Autodesk Fusion 360 part; units mm, degrees
sketch "Esquisse1" plane through (0, 0, 0) normal (0, 1, 0) x (1, 0, 0)
  line L0 (-367.4671, -125) -> (350, -125) construction
  arc A0 (209.2489, -218.6842) -> (223.8346, -225) centre (223.8346, -205) ccw
  arc A1 (-223.8346, -225) -> (-209.2489, -218.6842) centre (-223.8346, -205) ccw
  arc A2 (209.2489, -218.6842) -> (-209.2489, -218.6842) centre (0, -415) ccw
  line L1 (-305, 225) -> (305, 225)
  line L2 (325, 205) -> (325, -205)
  line L3 (305, -225) -> (223.8346, -225)
  line L4 (-325, -205) -> (-325, 205)
  arc A3 (325, 205) -> (305, 225) centre (305, 205) ccw
  line L5 (325, 225) -> (-325, -225) construction
  arc A4 (-305, 225) -> (-325, 205) centre (-305, 205) ccw
  arc A5 (-325, -205) -> (-305, -225) centre (-305, -205) ccw
  line L6 (-305, -225) -> (-223.8346, -225)
  line L7 (-325, 225) -> (325, -225) construction
  arc A6 (305, -225) -> (325, -205) centre (305, -205) ccw
  line L8 (215, -225) -> (325, -225)
  point P0 (-215, -225)
  dimension "d12" = 650
  dimension "d13" = 450
  dimension "d14" = 110
  dimension "d15" = 110
  dimension "d16" = 100
  dimension "d20" = 190
  dimension "d21" = 20
extrude "Extrusion1" add sketch "Esquisse1" along normal blind 3
sketch "Esquisse2" plane through (0, 3, 0) normal (0, 1, 0) x (-1, 0, 0)
  arc A0 (325, 205) -> (305, 225) centre (305, 205) ccw
  line L0 (305, 225) -> (223.8346, 225)
  arc A1 (223.8346, 225) -> (209.2489, 218.6842) centre (223.8346, 205) ccw
  arc A2 (-209.2489, 218.6842) -> (209.2489, 218.6842) centre (0, 415) ccw
  arc A3 (-209.2489, 218.6842) -> (-223.8346, 225) centre (-223.8346, 205) ccw
  line L1 (-223.8346, 225) -> (-305, 225)
  arc A4 (-305, 225) -> (-325, 205) centre (-305, 205) ccw
  line L2 (-325, 205) -> (-325, -205)
  arc A5 (-325, -205) -> (-305, -225) centre (-305, -205) ccw
  line L3 (-305, -225) -> (305, -225)
  arc A6 (305, -225) -> (325, -205) centre (305, -205) ccw
  line L4 (325, -205) -> (325, 205)
  line L5 (14.7224, 11.5) -> (0, 37)
  line L6 (-14.7224, 11.5) -> (14.7224, 11.5)
  line L7 (0, 37) -> (-14.7224, 11.5)
  line L8 (-61.5, -59.7224) -> (-61.5, -30.2776)
  line L9 (-87, -45) -> (-61.5, -59.7224)
  line L10 (-61.5, -30.2776) -> (-87, -45)
  line L11 (-14.7224, -101.5) -> (0, -127)
  line L12 (0, -127) -> (14.7224, -101.5)
  line L13 (14.7224, -101.5) -> (-14.7224, -101.5)
  line L14 (61.5, -30.2776) -> (61.5, -59.7224)
  line L15 (388.9907, -50) -> (-400, -50) construction
  line L16 (87, -45) -> (61.5, -30.2776)
  line L17 (61.5, -59.7224) -> (87, -45)
  point P0 (70, -45)
  point P1 (0, -110)
  point P2 (0, 20)
  dimension "d46" = 5
  dimension "d48" = 70
  dimension "d52" = 17
extrude "Extrusion2" cut sketch "Esquisse2" against normal blind 1 contours L5 L6 L7 | L8 L9 L10 | L11 L12 L13 | L14 L16 L17
sketch "Esquisse3" plane through (0, 3, 0) normal (0, 1, 0) x (-1, 0, 0)
  line L0 (0, -127) -> (-14.7224, -101.5)
  line L1 (-14.7224, -101.5) -> (14.7224, -101.5)
  line L2 (14.7224, -101.5) -> (0, -127)
  line L3 (-61.5, -59.7224) -> (-87, -45)
  line L4 (-87, -45) -> (-61.5, -30.2776)
  line L5 (-61.5, -30.2776) -> (-61.5, -59.7224)
  line L6 (61.5, -30.2776) -> (87, -45)
  line L7 (87, -45) -> (61.5, -59.7224)
  line L8 (61.5, -59.7224) -> (61.5, -30.2776)
  line L9 (14.7224, 11.5) -> (-14.7224, 11.5)
  line L10 (-14.7224, 11.5) -> (0, 37)
  line L11 (0, 37) -> (14.7224, 11.5)
  arc A0 (325, 205) -> (305, 225) centre (305, 205) ccw
  line L12 (305, 225) -> (223.8346, 225)
  arc A1 (223.8346, 225) -> (209.2489, 218.6842) centre (223.8346, 205) ccw
  arc A2 (-209.2489, 218.6842) -> (209.2489, 218.6842) centre (0, 415) ccw
  arc A3 (-209.2489, 218.6842) -> (-223.8346, 225) centre (-223.8346, 205) ccw
  line L13 (-223.8346, 225) -> (-305, 225)
  arc A4 (-305, 225) -> (-325, 205) centre (-305, 205) ccw
  line L14 (-325, 205) -> (-325, -205)
  arc A5 (-325, -205) -> (-305, -225) centre (-305, -205) ccw
  line L15 (-305, -225) -> (305, -225)
  arc A6 (305, -225) -> (325, -205) centre (305, -205) ccw
  line L16 (325, -205) -> (325, 205)
  line L17 (0, -325) -> (0, 225)
  line L18 (290, -225) -> (255, -260)
  line L19 (255, -260) -> (0, -260)
  line L20 (325, -175) -> (360, -140)
  line L21 (360, -140) -> (360, 140)
  line L22 (360, 140) -> (325, 175)
  line L23 (-255, -260) -> (0, -260)
  line L24 (-290, -225) -> (-255, -260)
  line L25 (-325, -175) -> (-360, -140)
  line L26 (-360, -140) -> (-360, 140)
  line L27 (-360, 140) -> (-325, 175)
  dimension "d22" = 35
  dimension "d23" = 45
  dimension "d24" = 580
  dimension "d25" = 35
  dimension "d26" = 45
  dimension "d27" = 45
  dimension "d28" = 350
  dimension "d30" = 30
extrude "Extrusion3" add sketch "Esquisse3" against normal up to surface (3 mm away) contours L15 L17 L23 L24 | L15 L17 L18 L19 | L14 L25 L26 L27 | L16 L20 L21 L22
sketch "Esquisse4" plane through (0, 3, 0) normal (0, 1, 0) x (-1, 0, 0)
  line L0 (0, -127) -> (-14.7224, -101.5)
  line L1 (-14.7224, -101.5) -> (14.7224, -101.5)
  line L2 (14.7224, -101.5) -> (0, -127)
  line L3 (-61.5, -59.7224) -> (-87, -45)
  line L4 (-87, -45) -> (-61.5, -30.2776)
  line L5 (-61.5, -30.2776) -> (-61.5, -59.7224)
  line L6 (61.5, -30.2776) -> (87, -45)
  line L7 (87, -45) -> (61.5, -59.7224)
  line L8 (61.5, -59.7224) -> (61.5, -30.2776)
  line L9 (14.7224, 11.5) -> (-14.7224, 11.5)
  line L10 (-14.7224, 11.5) -> (0, 37)
  line L11 (0, 37) -> (14.7224, 11.5)
  arc A0 (325, 205) -> (305, 225) centre (305, 205) ccw
  line L12 (305, 225) -> (223.8346, 225)
  arc A1 (223.8346, 225) -> (209.2489, 218.6842) centre (223.8346, 205) ccw
  arc A2 (-209.2489, 218.6842) -> (209.2489, 218.6842) centre (0, 415) ccw
  arc A3 (-209.2489, 218.6842) -> (-223.8346, 225) centre (-223.8346, 205) ccw
  line L13 (-223.8346, 225) -> (-305, 225)
  arc A4 (-305, 225) -> (-325, 205) centre (-305, 205) ccw
  line L14 (-325, 205) -> (-325, 175)
  line L15 (-325, 175) -> (-360, 140)
  line L16 (-360, 140) -> (-360, -140)
  line L17 (-360, -140) -> (-325, -175)
  line L18 (-325, -175) -> (-325, -205)
  arc A5 (-325, -205) -> (-305, -225) centre (-305, -205) ccw
  line L19 (-305, -225) -> (-290, -225)
  line L20 (-290, -225) -> (-255, -260)
  line L21 (-255, -260) -> (255, -260)
  line L22 (255, -260) -> (290, -225)
  line L23 (290, -225) -> (305, -225)
  arc A6 (305, -225) -> (325, -205) centre (305, -205) ccw
  line L24 (325, -205) -> (325, -175)
  line L25 (325, -175) -> (360, -140)
  line L26 (360, -140) -> (360, 140)
  line L27 (360, 140) -> (325, 175)
  line L28 (325, 175) -> (325, 205)
The listing builds one solid part. Answer for the finished solid, in the listing's coordinates (mm). A direction names the side the tool comes from. Coordinates: 2 decimals unless noted, no trailing zeros. Order: outer loops, then holes, each group sorted by start corner. A loop starts at its lowest first (then second) coordinate and runs counter-clockwise, first axis right, second up. Notation, with made-up numbers: M 13.5,68.25 L 62.5,68.25 A26 ccw 62.5,95.25 Z; hole C 24.25,41 d4. An arc over 180 degrees is marked long. Use CSV: the item, a comma, the result in double quotes.
Q1. A tool of negligible diameter and unlimited length cuts with its end or side. For faces 1 (the flat face through (-71, 2, -45)), 2 (the flat face through (342, 2, -158)), from which of +Z, -Z, +X, -X, +Y, -Y can it reach the whole face along a straight path? Write none if from no direction.
Here are the results:
face 1,"+Y"
face 2,"-Z, +X, +Y, -Y"
Q2. Section A-A (y = 0.6) is taken. Determine the outline of the cut face in (x, z).
Here are the results:
outline,"M -360,-140 L -325,-175 L -325,-205 A20 ccw -305,-225 L -290,-225 L -255,-260 L 255,-260 L 290,-225 L 305,-225 A20 ccw 325,-205 L 325,-175 L 360,-140 L 360,140 L 325,175 L 325,205 A20 ccw 305,225 L 223.83,225 A20 ccw 209.25,218.68 A286.92 cw -209.25,218.68 A20 ccw -223.83,225 L -305,225 A20 ccw -325,205 L -325,175 L -360,140 Z"
Q3. Determine the mould class of faces 3 (the flat face through (0, 2, 22)), 4 (the flat face through (-273, 2, -242)), 5 (the flat face through (273, 2, -242)), 6 (the flat face through (-5, 3, -21)) for opening direction X: pulls with the +X half, pulls with the -X half, needs draft (parallel to the pull), parting line crosses it, or undercut.
Here are the results:
face 3,"undercut"
face 4,"pulls with the -X half"
face 5,"pulls with the +X half"
face 6,"needs draft"
Q4. Section B-B (z = 151) is taken. Determine the outline of the cut face in (x, y).
Here are the results:
outline,"M -349,0 L -112.38,0 L -112.38,3 L -349,3 Z; M 112.38,0 L 349,0 L 349,3 L 112.38,3 Z"
Q5. Section D-D (x = -161) is taken. Determine the outline of the cut face in (y, z).
Here are the results:
outline,"M 0,-260 L 3,-260 L 3,177.5 L 0,177.5 Z"
Q6. Straight lines are drawn through the part: L1, parallel to X at y = 1.5, z = 198.5; L2, parallel to Z at x = 301.5, y = 2; L3, parallel to X at y = 2.5, z = -179. For each, find the intervals that lie inside material, in ascending order.
Here are the results:
L1,"-325 to -188.29, 188.29 to 325"
L2,"-225 to 225"
L3,"-325 to 325"
Q7. Given pin 1 Ø13 at (x, z) = (73.5, -50.5) entering from +Y; pin 2 Ø0.9 at (x, y) = (-294.5, 1) entering from -Z; pin 3 Ø1 at (y, z) = (0.5, -172) entering from +X; pin 4 Ø0.9 at (y, z) = (1, -187.5) entering from -X, each flat-ended and moving along its own axis, determine where each tip first touches the part or whether it passes through.
Here are the results:
pin 1,"y = 3"
pin 2,"z = -225"
pin 3,"x = 328.5"
pin 4,"x = -325"
Q8. Section C-C (x = 105.5) is taken. Determine the outline of the cut face in (y, z), then the cut area to 3 significant figures.
Here are the results:
outline,"M 0,-260 L 3,-260 L 3,148.18 L 0,148.18 Z"
area,"1,220 mm2"
